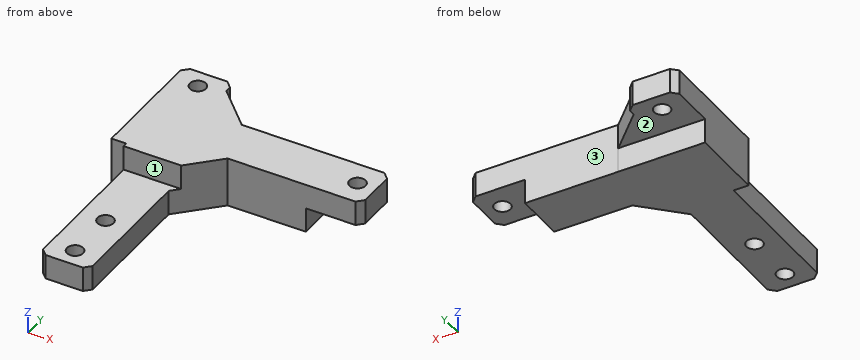
```python
from build123d import *

# Parameters (mm, degrees)
SKETCH_1_R          = 0.65
EXTRUDE_1_DEPTH     = 4
CUT_EXTRUDE_START   = -2
SKETCH_2_W          = 4
SKETCH_2_H          = 11.631287185
SKETCH_2_R          = 0.65
CUT_EXTRUDE_1_DEPTH = 2
SKETCH_3_W          = 4.48994314
SKETCH_3_H          = 4
SKETCH_3_R          = 0.65
SKETCH_3_W_2        = 4
SKETCH_3_H_2        = 3.998874997
CUT_EXTRUDE_2_DEPTH = 2
CHAMFER_1_SIZE      = 3
CHAMFER_2_SIZE      = 0.5


with BuildPart() as part:
    # 草图1 → 凸台-拉伸1 (new body)
    with BuildSketch(Plane.XY):
        Polygon((-4.3, -2.5), (9.5, -2.5), (9.5, 1.5), (-5.5, 1.5), (-5.5, 5.5), (-9.5, 5.5), (-9.5, 1.5), (-9.5, -4.5), (-8.3, -4.5), (-8.3, -16.5), (-4.3, -16.5), align=None)
        with Locations((8, -0.5)):
            Circle(SKETCH_1_R, mode=Mode.SUBTRACT)
        with Locations((-7.5, 4)):
            Circle(SKETCH_1_R, mode=Mode.SUBTRACT)
        with Locations((-6.3, -15)):
            Circle(SKETCH_1_R, mode=Mode.SUBTRACT)
        with Locations((-6.3, -10.8)):
            Circle(SKETCH_1_R, mode=Mode.SUBTRACT)
    extrude(amount=EXTRUDE_1_DEPTH)

    # 草图2 → 切除-拉伸1 (cut)
    with BuildSketch(Plane.XY.offset(4).offset(CUT_EXTRUDE_START)):
        with Locations((-6.3, -10.684356408)):
            Rectangle(SKETCH_2_W, SKETCH_2_H)
        with Locations((-6.3, -15)):
            Circle(SKETCH_2_R, mode=Mode.SUBTRACT)
        with Locations((-6.3, -10.8)):
            Circle(SKETCH_2_R, mode=Mode.SUBTRACT)
    extrude(amount=CUT_EXTRUDE_1_DEPTH, mode=Mode.SUBTRACT)

    # 草图3 → 切除-拉伸2 (cut)
    # profile 1 of 2: a face of its own
    with BuildSketch(Plane(origin=(0, 0, 0), x_dir=(-1, 0, 0), z_dir=(0, 0, -1))):
        with Locations((-7.25502843, -0.5)):
            Rectangle(SKETCH_3_W, SKETCH_3_H)
        with Locations((-8, -0.5)):
            Circle(SKETCH_3_R, mode=Mode.SUBTRACT)
    # profile 2 of 2: a face of its own
    with BuildSketch(Plane(origin=(0, 0, 0), x_dir=(-1, 0, 0), z_dir=(0, 0, -1))):
        with Locations((7.5, 3.500562502)):
            Rectangle(SKETCH_3_W_2, SKETCH_3_H_2)
        with Locations((7.5, 4)):
            Circle(SKETCH_3_R, mode=Mode.SUBTRACT)
    extrude(amount=-CUT_EXTRUDE_2_DEPTH, mode=Mode.SUBTRACT)

    # 倒角1
    chamfer_1_edges = [part.edges().sort_by_distance(p)[0] for p in [
        (-4.3, -2.5, 2),
        (-5.5, 1.5, 2),
    ]]
    chamfer(chamfer_1_edges, length=CHAMFER_1_SIZE)

    # 倒角2
    chamfer_2_edges = [part.edges().sort_by_distance(p)[0] for p in [
        (9.5, -2.5, 3),
        (-9.5, 5.5, 3),
        (-5.5, 5.5, 3),
        (9.5, 1.5, 3),
        (-4.3, -16.5, 1),
        (-8.3, -16.5, 1),
    ]]
    chamfer(chamfer_2_edges, length=CHAMFER_2_SIZE)


solid = part.part
```
Check sheet for the modelled part. Datum: model origin and axes. Units: mm. Face numbers are marked on the shaded views. A direction names the side the tool comes from. Round coordinates to 2 decimals unless told otherwise and drop trailing zeros. Write each loop counter-clockwise with the first axis right and the second up, starting at its lowest first coordinate (ties: lowest second). Pieces come first, ordered by that corner, then holes. Notation, with made-up numbers: (84, 73.5) -> (123, 73.5) arc R21 ccw to (123, 82.5) -> close; hole circle Ø10 at (-0.5, 78). An arc over 180 degrees is marked (long way). One line per question, with ' | ' between items. Start each with the question number.
1. Sectioned sample at D-D, the plane y = -0.5. Record the cut outline in (x, z).
2. Sectioned sample at B-B, the plane z = 3.2. Record the cut outline in (x, y).
3. Sectioned sample at A-A, the plane x = 8. Record the cut outline in (y, z).
4. Scan lines: line 1 along Y through (x, z) = (-6.3, 1.15); line 2 along Y through (x, z) = (8, 2.5); line 3 along Y through (x, z) = (-8.5, 0.35). Record each from-to range of solid material in increasing order. Write a range as from..to.
5. Set-up check for the marked faces 1, 2 and 3: record each of +Z, -Z, +X, -X, +Y, -Y from which the full face is reachable in a straight line by a thin tool's end or side.
6. Depth check by flat-ended pin: pin 1 (1.7 mm diameter, centred on x = -6.3, y = -15, fed in from -Z); pin 2 (2 mm diameter, centred on x = 2, z = 3, fed in from -Y); pin 3 (1.6 mm diameter, centred on y = -12.5, z = 1, fed in from +X); pin 4 (1.4 mm diameter, centred on x = -6, y = -13, fed in from +Z). Enter the tip coordinate at first touch or a pass-through.
7. Sectioned sample at C-C, the plane x = -6.3. Record the cut outline in (y, z), then the cut area to 3 significant figures.
Taken from the geometry:
1) outline: (-9.5, 0) -> (5.01, 0) -> (5.01, 2) -> (7.35, 2) -> (7.35, 4) -> (-9.5, 4) -> close; (8.65, 2) -> (9.5, 2) -> (9.5, 4) -> (8.65, 4) -> close
2) outline: (-9.5, -4.5) -> (-8.3, -4.5) -> (-8.3, -4.87) -> (-3.67, -4.87) -> (-1.3, -2.5) -> (9, -2.5) -> (9.5, -2) -> (9.5, 1) -> (9, 1.5) -> (-2.5, 1.5) -> (-5.5, 4.5) -> (-5.5, 5) -> (-6, 5.5) -> (-9, 5.5) -> (-9.5, 5) -> close; hole circle Ø1.3 at (-7.5, 4); hole circle Ø1.3 at (8, -0.5)
3) outline: (-2.5, 2) -> (-1.15, 2) -> (-1.15, 4) -> (-2.5, 4) -> close; (0.15, 2) -> (1.5, 2) -> (1.5, 4) -> (0.15, 4) -> close
4) line 1: y = -16.5..-15.65, -14.35..-11.45, -10.15..1.5 | line 2: y = -2.5..-1.15, 0.15..1.5 | line 3: y = -4.5..1.5
5) face 1: +Z, +X, -X, -Y | face 2: -Z, +X, -X, +Y | face 3: +Z, -Z, +X, +Y
6) pin 1: stops at z = 0 | pin 2: stops at y = -2.5 | pin 3: stops at x = -4.3 | pin 4: stops at z = 2
7) outline: (-16.5, 0) -> (-15.65, 0) -> (-15.65, 2) -> (-16.5, 2) -> close; (-14.35, 0) -> (-11.45, 0) -> (-11.45, 2) -> (-14.35, 2) -> close; (-10.15, 0) -> (1.5, 0) -> (1.5, 2) -> (5.5, 2) -> (5.5, 4) -> (-4.87, 4) -> (-4.87, 2) -> (-10.15, 2) -> close | area: 51.5 mm^2
